Design review of the part built by this model. Coordinates are the model's own, in mm. Coordinates: 2 decimals unless noted, no trailing zeros. Write each loop counter-clockwise with the first axis right and the second up, starting at its lowest first coordinate (ties: lowest second). Pieces come first, ordered by that corner, then holes.
Q1. The part is to be moulded in two halves that separate along Z. For faces 1 (the face through (40.53, -40.56, -19.79)), 2 (the face through (-3.252, -50.42, -10.337)), 3 (the face through (0, -20, 5)), 4 (the face through (-36.542, -40.56, 27.282)), say which applies: +Z half, -Z half, draft (parallel to the pull), parting line (faces both ways), or undercut.
Q2. Add section B-B, the plane x = 0. Give the boundary of the cut face in (y, z), plus the area to 3 significant figures.
Q3. Add section C-C, the plane z = 8. Give the boundary of the cut face in (x, y), plus the area to 3 significant figures.
Q4. Clearance check with a flat-ended pin moving along its axis: pin 1 Ø15 at (x, z) = (4, 4) entering from -Y. State where the tip first meets the part, or that it passes through.
Q5. To check wall thickness, follow probe 1 along Z at (x, y) = (0, -47); probe 2 along X at (y, z) = (-58.5, 9); probe 3 along X at (y, z) = (-66, -8). State the ranges of each line that lie inside material, in increasing order.
Q6. Add section A-A, the plane y = -39. Give the boundary of the cut face in (x, z), plus the area to 3 significant figures.
from build123d import *

# Parameters (mm, degrees)
F0_W     = 80
F0_H     = 50
F1_DEPTH = 80
F2_R     = 15
F3_DEPTH = 60
F4_R     = 5


with BuildPart() as f1:
    # F0 (on Front) → F1 (new body)
    with BuildSketch(Plane.XZ):
        with Locations((2.032589, 3.78601)):
            Rectangle(F0_W, F0_H)
    extrude(amount=F1_DEPTH)

    # F2 (on face) → F3 (cut)
    with BuildSketch(Plane.XZ.offset(80)):
        with Locations((0, 4.305844)):
            Circle(F2_R)
    extrude(amount=-F3_DEPTH, mode=Mode.SUBTRACT)

    # F4
    f4_edges = [f1.edges().sort_by_distance(p)[0] for p in [
        (-37.967411, -40, 28.78601),
        (42.032589, -40, 28.78601),
        (-37.967411, -40, -21.21399),
        (42.032589, -40, -21.21399),
    ]]
    fillet(f4_edges, radius=F4_R)


solid = f1.part
Here are the results:
1. face 1: -Z half
1. face 2: undercut
1. face 3: undercut
1. face 4: +Z half
2. outline: (-80, -21.21) - (0, -21.21) - (0, 28.79) - (-80, 28.79) - (-80, 19.31) - (-20, 19.31) - (-20, -10.69) - (-80, -10.69) - close
2. area: 2,200 mm2
3. outline: (-37.97, -80) - (-14.54, -80) - (-14.54, -20) - (14.54, -20) - (14.54, -80) - (42.03, -80) - (42.03, 0) - (-37.97, 0) - close
3. area: 4,660 mm2
4. pin 1: stops at y = -20
5. probe 1: z = -21.21 to -10.69, 19.31 to 28.79
5. probe 2: x = -37.97 to -14.25, 14.25 to 42.03
5. probe 3: x = -37.97 to -8.58, 8.58 to 42.03
6. outline: (-37.97, -16.21) arc R5 ccw to (-32.97, -21.21) - (37.03, -21.21) arc R5 ccw to (42.03, -16.21) - (42.03, 23.79) arc R5 ccw to (37.03, 28.79) - (-32.97, 28.79) arc R5 ccw to (-37.97, 23.79) - close; hole circle Ø30 at (0, 4.31)
6. area: 3,270 mm2
